Could you check a few things on this model? Use its own coordinates, in mm. Face numbers are marked on the shaded views. A direction names the side the tool comes from. Round coordinates to 2 decimals unless told otherwise and drop trailing zeros. Write each loop counter-clockwise with the first axis right and the second up, starting at its lowest first coordinate (ties: lowest second). Pieces come first, ordered by that corner, then holes.
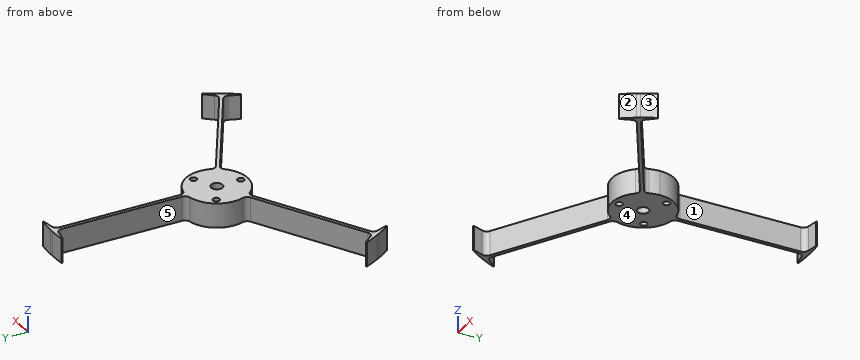
```python
from build123d import *

# Parameters (mm, degrees)
F0_R     = 1.5875
F0_R_2   = 2.677996
F1_DEPTH = 11.43
F2_R     = 0.254
F3_R     = 2.54


with BuildPart() as f1:
    # F0 (on Top) → F1 (new body)
    with BuildSketch(Plane.XY):
        with BuildLine():
            ThreePointArc((14.5, 0), (10.540867, 9.956913), (0.8255, 14.476483))
            ThreePointArc((0.8255, 14.476483), (0, 14.5), (-0.8255, 14.476483))
            ThreePointArc((-0.8255, 14.476483), (-12.557368, 7.25), (-12.949752, -6.523337))
            ThreePointArc((-12.949752, -6.523337), (-12.557368, -7.25), (-12.124252, -7.953145))
            ThreePointArc((-12.124252, -7.953145), (0, -14.5), (12.124252, -7.953145))
            ThreePointArc((12.124252, -7.953145), (12.557368, -7.25), (12.949752, -6.523337))
            ThreePointArc((12.949752, -6.523337), (14.107115, -3.352507), (14.5, 0))
        make_face()
        with Locations((0, -11.226573)):
            Circle(F0_R, mode=Mode.SUBTRACT)
        with Locations((-9.722497, 5.613286)):
            Circle(F0_R, mode=Mode.SUBTRACT)
        Circle(F0_R_2, mode=Mode.SUBTRACT)
        with Locations((9.722497, 5.613286)):
            Circle(F0_R, mode=Mode.SUBTRACT)
        with BuildLine():
            Line((0.8255, 75.331596), (0.8255, 77.465602))
            ThreePointArc((0.8255, 77.465602), (0, 77.47), (-0.8255, 77.465602))
            Line((-0.8255, 77.465602), (-0.8255, 75.331596))
            Line((-0.8255, 75.331596), (-0.8255, 14.476483))
            ThreePointArc((-0.8255, 14.476483), (0, 14.5), (0.8255, 14.476483))
            Line((0.8255, 14.476483), (0.8255, 75.331596))
        make_face()
        with BuildLine():
            ThreePointArc((-12.124252, -7.953145), (-12.557368, -7.25), (-12.949752, -6.523337))
            Line((-12.949752, -6.523337), (-65.651826, -36.950894))
            Line((-65.651826, -36.950894), (-67.499929, -38.017897))
            ThreePointArc((-67.499929, -38.017897), (-67.090988, -38.735), (-66.674429, -39.447705))
            Line((-66.674429, -39.447705), (-64.826326, -38.380702))
            Line((-64.826326, -38.380702), (-12.124252, -7.953145))
        make_face()
        with BuildLine():
            ThreePointArc((66.674429, -39.447705), (67.090988, -38.735), (67.499929, -38.017897))
            Line((67.499929, -38.017897), (65.651826, -36.950894))
            Line((65.651826, -36.950894), (12.949752, -6.523337))
            ThreePointArc((12.949752, -6.523337), (12.557368, -7.25), (12.124252, -7.953145))
            Line((12.124252, -7.953145), (64.826326, -38.380702))
            Line((64.826326, -38.380702), (66.674429, -39.447705))
        make_face()
        with BuildLine():
            Line((-0.8255, 75.331596), (-0.8255, 77.465602))
            ThreePointArc((-0.8255, 77.465602), (-5.211335, 77.29452), (-9.580441, 76.875328))
            Line((-9.580441, 76.875328), (-0.8255, 75.331596))
        make_face()
        with BuildLine():
            Line((0.8255, 75.331596), (9.580441, 76.875328))
            ThreePointArc((9.580441, 76.875328), (5.211335, 77.29452), (0.8255, 77.465602))
            Line((0.8255, 77.465602), (0.8255, 75.331596))
        make_face()
        with BuildLine():
            ThreePointArc((61.785766, -46.734569), (64.333351, -43.160408), (66.674429, -39.447705))
            Line((66.674429, -39.447705), (64.826326, -38.380702))
            Line((64.826326, -38.380702), (61.785766, -46.734569))
        make_face()
        with BuildLine():
            ThreePointArc((67.499929, -38.017897), (69.544686, -34.134112), (71.366207, -30.140759))
            Line((71.366207, -30.140759), (65.651826, -36.950894))
            Line((65.651826, -36.950894), (67.499929, -38.017897))
        make_face()
        with BuildLine():
            ThreePointArc((-66.674429, -39.447705), (-64.333351, -43.160408), (-61.785766, -46.734569))
            Line((-61.785766, -46.734569), (-64.826326, -38.380702))
            Line((-64.826326, -38.380702), (-66.674429, -39.447705))
        make_face()
        with BuildLine():
            Line((-65.651826, -36.950894), (-71.366207, -30.140759))
            ThreePointArc((-71.366207, -30.140759), (-69.544686, -34.134112), (-67.499929, -38.017897))
            Line((-67.499929, -38.017897), (-65.651826, -36.950894))
        make_face()
    extrude(amount=F1_DEPTH)

    # F2
    f2_edges = [f1.edges().sort_by_distance(p)[0] for p in [
        (71.366207, -30.140759, 5.715),
        (61.785766, -46.734569, 5.715),
        (-71.366207, -30.140759, 5.715),
        (-61.785766, -46.734569, 5.715),
        (-9.580441, 76.875328, 5.715),
        (9.580441, 76.875328, 5.715),
    ]]
    fillet(f2_edges, radius=F2_R)

    # F3
    f3_edges = [f1.edges().sort_by_distance(p)[0] for p in [
        (-12.124252, -7.953145, 5.715),
        (-12.949752, -6.523337, 5.715),
        (-0.8255, 14.476483, 5.715),
        (0.8255, 14.476483, 5.715),
        (12.949752, -6.523337, 5.715),
        (12.124252, -7.953145, 5.715),
        (-64.826326, -38.380702, 5.715),
        (-65.651826, -36.950894, 5.715),
        (-0.8255, 75.331596, 5.715),
        (64.826326, -38.380702, 5.715),
        (65.651826, -36.950894, 5.715),
        (0.8255, 75.331596, 5.715),
    ]]
    fillet(f3_edges, radius=F3_R)


solid = f1.part
```
Q1. Imagine slicing it at A-A, the plane y = -21.5. Write out the boundary of the cut face in (x, z).
Q2. If I drill on L1, parallel to Y at x = 0, z = 5.25; L2, parallel to X at y = -10, z = 7.5; L3, parallel to X at y = 32.5, z = 6.75, over which ranges is the centre line in solid material (lowest first)?
Q3. Imagine slicing it at D-D, the plane x = 56.5. Write out the boundary of the cut face in (y, z).
Q4. On a 3-axis mill with a long thin cutter (end or side, diameter ignored), from which of +Z, -Z, +X, -X, +Y, -Y can I reach the whole of each face in a straight line? I mean the marked faces 1 and 2. Say none if no direction works.
Q5. Imagine slicing it at C-C, the plane y = 66. Write out the boundary of the cut face in (x, z), then the cut area to 3 significant figures.
Q6. Imagine slicing it at B-B, the plane z = 2.75. Count the separate pieces of the cut face and the enclosed holes in it, then the cut area to 3 significant figures.
Q7. We'd pull the mould along Y, two halves only. Please class the marked faces 3, 4 and 5: pulls with the +Y half, pulls with the -Y half, needs draft (parallel to the pull), parting line crosses it, or undercut.
Q8. I'm going to push flat-ended pins straight in: pin 1 Ø5.5 at (y, z) = (36.5, 5.5) entering from +X; pin 2 Ø1 at (x, z) = (-54, 9.5) entering from -Y. Where does each tip first touch, or does it pass through?
Results found:
1. outline: (-38.89, 0) - (-35.59, 0) - (-35.59, 11.43) - (-38.89, 11.43) - close; (35.59, 0) - (38.89, 0) - (38.89, 11.43) - (35.59, 11.43) - close
2. L1: y = -14.5 to -12.81, -9.64 to -2.68, 2.68 to 77.47
2. L2: x = -18.97 to -15.67, -10.5 to -1.01, 1.01 to 10.5, 15.67 to 18.97
2. L3: x = -0.83 to 0.83
3. outline: (-33.57, 0) - (-31.67, 0) - (-31.67, 11.43) - (-33.57, 11.43) - close
4. face 1: +Z, -Z, +X
4. face 2: +Z, -Z, +X, -Y
5. outline: (-0.83, 0) - (0.83, 0) - (0.83, 11.43) - (-0.83, 11.43) - close
5. area: 18.9 mm2
6. separate pieces: 1
6. enclosed holes: 4
6. area: 996 mm2
7. face 3: pulls with the -Y half
7. face 4: needs draft
7. face 5: undercut
8. pin 1: stops at x = 0.83
8. pin 2: stops at y = -32.42
